The listing builds one solid part. Answer for the finished solid, in the listing's coordinates (mm). Give positions to 0.01 mm unless a question says otherwise; leave off trailing zeros. Write each loop counter-clockwise with the first axis right and the second up, starting at its lowest first coordinate (ties: lowest second). Pieces come first, ordered by that corner, then holes. Notation, with made-up numbers: (-14.5, -4) - (-7.5, -4) arc R16 ccw to (-7.5, 22) - close; hole circle Ø4 at (18, -33). An arc over 180 degrees is marked (long way). One line per question, with ' | ' between items. Start each with the question number.
1. A cutting plane is placed at A-A (z = 21). Determine the outline of the cut face in (x, y).
2. A cutting plane is placed at B-B (y = 1.1). State how many separate pieces and enclosed holes the cut face has, then the cut area to 3 significant figures.
3. Find the intervals of material crossed by L1, parallel to Z at x = 67.1, y = 1.25; L2, parallel to X at y = 2.25, z = -92.7; L3, parallel to X at y = 3.2, z = 93.1, in increasing order. Write a range as from..to.
4. Given P1, Ø4, axis at x = -66.28, z = 93.1, coming from the +Y side; P2, Ø1.8, axis at x = 22.6, z = 12.16, coming from the -Y side, each flat-ended and moving along its own axis, determine where each tip first touches the part or whether it passes through.
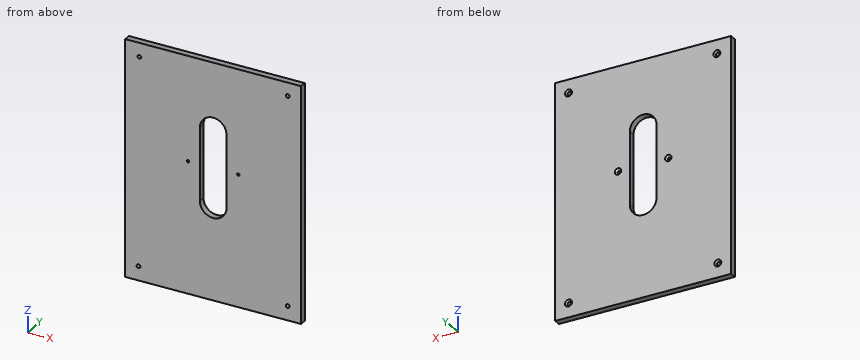
```python
from build123d import *

# Parameters (mm, degrees)
SKETCH1_W                                       = 158
SKETCH1_H                                       = 210.8
BOSS_EXTRUDE1_DEPTH                             = 5.9
CSK_FOR_M3_FLAT_HEAD_MACHINE_SCREW1_D           = 3.4
CSK_FOR_M3_FLAT_HEAD_MACHINE_SCREW1_DEPTH       = 10
CSK_FOR_M3_FLAT_HEAD_MACHINE_SCREW1_CSINK_D     = 6.3
CSK_FOR_M3_FLAT_HEAD_MACHINE_SCREW1_CSINK_ANGLE = 90
CSK_FOR_M3_FLAT_HEAD_MACHINE_SCREW1_TIP         = 1.021463052
CUT_EXTRUDE1_DEPTH                              = 132.852076207
F_4_40_TAPPED_HOLE1_D                           = 2.2606
F_4_40_TAPPED_HOLE1_DEPTH                       = 10
F_4_40_TAPPED_HOLE1_CSINK_D                     = 5.715
F_4_40_TAPPED_HOLE1_CSINK_ANGLE                 = 100
F_4_40_TAPPED_HOLE1_TIP                         = 0.679152758


with BuildPart() as part:
    # Sketch1 → Boss-Extrude1 (new body)
    with BuildSketch(Plane(origin=(0, 0, 0), x_dir=(1, 0, 0), z_dir=(0, 1, 0))):
        Rectangle(SKETCH1_W, SKETCH1_H)
    extrude(amount=BOSS_EXTRUDE1_DEPTH)

    # CSK for M3 Flat Head Machine Screw1
    with Locations(Plane(origin=(0, 5.9, 0), x_dir=(1, 0, 0), z_dir=(0, 1, 0))):
        with Locations((67.1, 92.7), (67.1, -93.5), (-66.28397659, -93.1), (-67.1, 92.7)):
            CounterSinkHole(CSK_FOR_M3_FLAT_HEAD_MACHINE_SCREW1_D / 2, CSK_FOR_M3_FLAT_HEAD_MACHINE_SCREW1_CSINK_D / 2, depth=CSK_FOR_M3_FLAT_HEAD_MACHINE_SCREW1_DEPTH, counter_sink_angle=CSK_FOR_M3_FLAT_HEAD_MACHINE_SCREW1_CSINK_ANGLE)
            with Locations((0, 0, -(CSK_FOR_M3_FLAT_HEAD_MACHINE_SCREW1_DEPTH + CSK_FOR_M3_FLAT_HEAD_MACHINE_SCREW1_TIP / 2))):  # 118° drill point
                Cone(0, CSK_FOR_M3_FLAT_HEAD_MACHINE_SCREW1_D / 2, CSK_FOR_M3_FLAT_HEAD_MACHINE_SCREW1_TIP, mode=Mode.SUBTRACT)

    # Sketch4 → Cut-Extrude1 (cut, through all)
    with BuildSketch(Plane(origin=(0, 5.9, 0), x_dir=(1, 0, 0), z_dir=(0, 1, 0))):
        with BuildLine():
            Line((-11.991361004, 20.34), (-11.991361004, -44.66))
            add(Edge.make_bspline(
                [(-11.991361004, -44.66), (-11.991361004, -68.642722008), (11.991361004, -68.642722008), (11.991361004, -44.66)],
                knots=[0, 0, 0, 0, 1, 1, 1, 1], degree=3, weights=[1, 0.333333333, 0.333333333, 1]))
            Line((11.991361004, -44.66), (11.991361004, 20.34))
            add(Edge.make_bspline(
                [(11.991361004, 20.34), (11.991361004, 44.322722008), (-11.991361004, 44.322722008), (-11.991361004, 20.34)],
                knots=[0, 0, 0, 0, 1, 1, 1, 1], degree=3, weights=[1, 0.333333333, 0.333333333, 1]))
        make_face()
    extrude(amount=-CUT_EXTRUDE1_DEPTH, mode=Mode.SUBTRACT)

    # #4-40 Tapped Hole1
    with Locations(Plane(origin=(0, 5.9, 0), x_dir=(1, 0, 0), z_dir=(0, 1, 0))):
        with Locations((-22.6, -12.16), (22.6, -12.16)):
            CounterSinkHole(F_4_40_TAPPED_HOLE1_D / 2, F_4_40_TAPPED_HOLE1_CSINK_D / 2, depth=F_4_40_TAPPED_HOLE1_DEPTH, counter_sink_angle=F_4_40_TAPPED_HOLE1_CSINK_ANGLE)
            with Locations((0, 0, -(F_4_40_TAPPED_HOLE1_DEPTH + F_4_40_TAPPED_HOLE1_TIP / 2))):  # 118° drill point
                Cone(0, F_4_40_TAPPED_HOLE1_D / 2, F_4_40_TAPPED_HOLE1_TIP, mode=Mode.SUBTRACT)


solid = part.part
```
Determined:
1) outline: (-79, 0) - (-11.99, 0) - (-11.99, 5.9) - (-79, 5.9) - close; (11.99, 0) - (79, 0) - (79, 5.9) - (11.99, 5.9) - close
2) separate pieces: 1 | enclosed holes: 7 | area: 31,300 mm2
3) L1: -105.4..-94.4, -91..91.8, 95.2..105.4 | L2: -79..-68.8, -65.4..65.4, 68.8..79 | L3: -79..-67.98, -64.58..65.45, 68.75..79
4) P1: y = 4.75 | P2: through
